Geometry: see drawing. Coordinates: mm, zero at the bounding-box minimum. A direction names the side the tool comes from. Coordinates: 2 decimals unless noted, no trailing zeros. Write each loop counter-clockwise with the first axis right and the second up, starting at its lowest first coordinate (ties: lowest second). Pieces come first, ordered by that corner, then holes. Notation, with made-up numbers: M -38,51 L -32,51 A11 ccw -32,67 Z; hole C 79.25,82.25 d2. An arc over 180 degrees is marked long. Write item = value, one per line. Start each with the question number.
1. Section query A-A (y = 31.5). Output: boundary loops of the cut face in (x, z).
2. Line query: line 1 along Z through (x, y) = (40, 4); line 2 along Y through (x, z) = (19, 20.75). Output: solid intervals per line, ascending.
3. Pull-direction query (Z, two-part tool) for the marked faces 3, 4, 5 and 6; classes: pulls with the +Z half, pulls with the -Z half, needs draft (parallel to the pull), parting line crosses it, or undercut.
4. Section query B-B (x = 33.5). Output: boundary loops of the cut face in (y, z), then the cut area to 3 significant figures.
5. Pin query (flat end, axial travel): pin 1 Ø3.5 at (x, z) = (2.5, 17) entering from +Y; pin 2 Ø6 at (x, z) = (36.5, 9.5) entering from +Y; pin 3 Ø1 at (y, z) = (2, 15.5) entering from +X. Return the tip coordinate at first contact, or that it passes through.
6. Access query for the marked faces 1 and 2. Directions: +Z, -Z, +X, -X, +Y, -Y. A direction counts if a zero-diameter tool reaches every point of the face in a straight line with its end or side. Return the directions, or none.
7. Section query D-D (z = 9). Output: boundary loops of the cut face in (x, y).
8. Section query C-C (y = 5). Output: boundary loops of the cut face in (x, z).
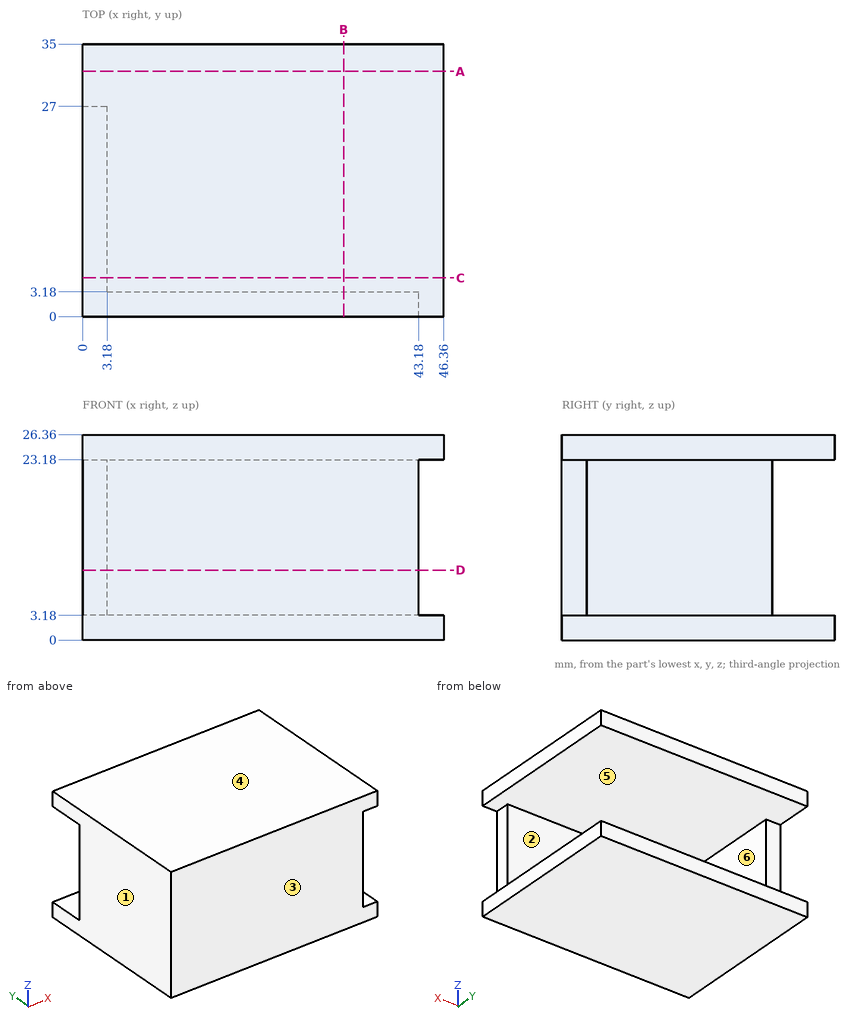
Results are:
q1.outline = M 0,0 L 46.36,0 L 46.36,3.18 L 0,3.18 Z; M 0,23.18 L 46.36,23.18 L 46.36,26.36 L 0,26.36 Z
q2.line_1 = 0 to 3.18, 23.18 to 26.36
q2.line_2 = 0 to 3.18
q3.face_3 = needs draft
q3.face_4 = pulls with the +Z half
q3.face_5 = undercut
q3.face_6 = undercut
q4.outline = M 0,0 L 35,0 L 35,3.18 L 3.18,3.18 L 3.18,23.18 L 35,23.18 L 35,26.36 L 0,26.36 Z
q4.area = 286 mm^2
q5.pin_1 = 27
q5.pin_2 = 3.18
q5.pin_3 = 43.18
q6.face_1 = +Z, -Z, -X, +Y, -Y
q6.face_2 = +X, +Y
q7.outline = M 0,0 L 43.18,0 L 43.18,3.18 L 3.18,3.18 L 3.18,27 L 0,27 Z
q8.outline = M 0,0 L 46.36,0 L 46.36,3.18 L 3.18,3.18 L 3.18,23.18 L 46.36,23.18 L 46.36,26.36 L 0,26.36 Z
